from build123d import *
from OCP.BRepFilletAPI import BRepFilletAPI_MakeFillet

# Parameters (mm, degrees)
SKETCH1_W           = 55
SKETCH1_H           = 30
BOSS_EXTRUDE1_DEPTH = 3
CUT_EXTRUDE1_DEPTH  = 32.468237955
SKETCH3_W           = 6.4
SKETCH3_H           = 2
CUT_EXTRUDE2_DEPTH  = 32.468237955
SKETCH4_W           = 20.5
SKETCH4_H           = 16
CUT_EXTRUDE3_DEPTH  = 32.468237955
FILLET1_R1          = 3
FILLET1_R2          = 2.5
FILLET1_R3          = 2


with BuildPart() as part:
    # Sketch1 → Boss-Extrude1 (new body)
    with BuildSketch(Plane(origin=(0, 0, 0), x_dir=(1, 0, 0), z_dir=(0, 1, 0))):
        Rectangle(SKETCH1_W, SKETCH1_H)
    extrude(amount=BOSS_EXTRUDE1_DEPTH)

    # Sketch2 → Cut-Extrude1 (cut, through all)
    with BuildSketch(Plane(origin=(0, 3, 0), x_dir=(1, 0, 0), z_dir=(0, 1, 0))):
        with BuildLine():
            Line((17, -5.5), (24, -5.5))
            ThreePointArc((24, -5.5), (26.5, -8), (24, -10.5))
            Line((24, -10.5), (17, -10.5))
            ThreePointArc((17, -10.5), (14.5, -8), (17, -5.5))
        make_face()
        with BuildLine():
            Line((-17, -5.5), (-24, -5.5))
            ThreePointArc((-24, -5.5), (-26.5, -8), (-24, -10.5))
            Line((-24, -10.5), (-17, -10.5))
            ThreePointArc((-17, -10.5), (-14.5, -8), (-17, -5.5))
        make_face()
        with BuildLine():
            Line((-2, -2), (-2, 8))
            ThreePointArc((-2, 8), (0, 10), (2, 8))
            Line((2, 8), (2, -2))
            ThreePointArc((2, -2), (0, -4), (-2, -2))
        make_face()
    extrude(amount=-CUT_EXTRUDE1_DEPTH, mode=Mode.SUBTRACT)

    # Sketch3 → Cut-Extrude2 (cut, through all)
    with BuildSketch(Plane(origin=(0, 3, 0), x_dir=(1, 0, 0), z_dir=(0, 1, 0))):
        with Locations((0, 15)):
            Rectangle(SKETCH3_W, SKETCH3_H)
    extrude(amount=-CUT_EXTRUDE2_DEPTH, mode=Mode.SUBTRACT)

    # Sketch4 → Cut-Extrude3 (cut, through all)
    with BuildSketch(Plane(origin=(0, 3, 0), x_dir=(1, 0, 0), z_dir=(0, 1, 0))):
        with Locations((-17.25, 7)):
            Rectangle(SKETCH4_W, SKETCH4_H)
        with Locations((17.25, 7)):
            Rectangle(SKETCH4_W, SKETCH4_H)
    extrude(amount=-CUT_EXTRUDE3_DEPTH, mode=Mode.SUBTRACT)

    # Fillet1: one fillet with a radius per group of edges: ONE call of the kernel's fillet builder (fillet() takes one radius for all edges)
    fillet1_edges_1 = [part.edges().sort_by_distance(p)[0] for p in [
        (7, 1.5, 1),
        (-7, 1.5, 1),
    ]]
    fillet1_edges_2 = [part.edges().sort_by_distance(p)[0] for p in [
        (-27.5, 1.5, 1),
        (-27.5, 1.5, 15),
    ]]
    fillet1_edges_3 = [part.edges().sort_by_distance(p)[0] for p in [
        (27.5, 1.5, 1),
        (27.5, 1.5, 15),
        (7, 1.5, -15),
        (-7, 1.5, -15),
    ]]
    fillet1 = BRepFilletAPI_MakeFillet(part.part.solid().wrapped)
    for e in fillet1_edges_1:
        fillet1.Add(FILLET1_R1, e.wrapped)
    for e in fillet1_edges_2:
        fillet1.Add(FILLET1_R2, e.wrapped)
    for e in fillet1_edges_3:
        fillet1.Add(FILLET1_R3, e.wrapped)
    add(Compound.cast(fillet1.Shape()), mode=Mode.REPLACE)


solid = part.part
Geometry check sheet. Reference: the model listing, model coordinates, mm. A direction names the side the tool comes from. Give positions to 0.01 mm unless a question says otherwise; leave off trailing zeros. Loops run counter-clockwise (first coordinate to the right, second up) from the corner with the lowest first, then second, coordinate; pieces in that order, holes last. Notation, with made-up numbers: M 37.5,49 L 44.5,49 A24 ccw 44.5,77 Z; hole C 67,30.5 d11. An arc over 180 degrees is marked long. Answer as a JSON object with one key per item and string values. Group by question number.
Item 1: Material ranges on L1, parallel to Z at x = 17, y = 1.5; L2, parallel to X at y = 1.2, z = 9; L3, parallel to X at y = 0.35, z = -12.5, recorded low to high.
Item 2: Access from +Z, -Z, +X, -X, +Y, -Y to the whole of each face (thin tool, end or side, straight path). Record for faces 4 (the flat face through (7, 2, -7)), 5 (the cylindrical face through (-27, 2, 14)), 6 (the flat face through (2, 2, -3)), 7 (the flat face through (-18, 2, 1)).
Item 3: Gauge pin test, flat ends, axial feed: pin 1 (0.8 mm diameter, centred on y = 1, z = -14.5, fed in from -X); pin 2 (0.9 mm diameter, centred on x = -15, y = 1, fed in from -Z); pin 3 (0.9 mm diameter, centred on y = 1, z = -2.5, fed in from +X). Record the tip position at first contact, or that the pin passes through.
Item 4: Sectioned sample at B-B on y = 0.6. Give the number of separate pieces and of enclosed holes in the cut face, plus the area to 3 significant figures.
Item 5: Sectioned sample at A-A on x = 20.5. Record the boundary of the cut face in (y, z).
Item 6: Mould release check, pull along X, two halves, no side actions. Record for faces 1 (the flat face through (0, 3, 6)), 2 (the flat face through (-2, 2, -3)), 3 (the cylindrical face through (26.9, 1.52, 14.43)): pulls with the +X half, pulls with the -X half, needs draft (parallel to the pull), parting line crosses it, or undercut.
Findings below:
{
 "1": {"L1": "1 to 5.5, 10.5 to 15", "L2": "-27.5 to -26.29, -14.71 to 14.71, 26.29 to 27.5", "L3": "-7 to 7"},
 "2": {"face 4": "-Z, +X, +Y, -Y", "face 5": "+Z, -X, +Y, -Y", "face 6": "+Y, -Y", "face 7": "-Z, -X, +Y, -Y"},
 "3": {"pin 1": "x = -6.67", "pin 2": "z = 1", "pin 3": "x = 7"},
 "4": {"separate pieces": "1", "enclosed holes": "3", "area": "824 mm2"},
 "5": {"outline": "M 0,1 L 3,1 L 3,5.5 L 0,5.5 Z; M 0,10.5 L 3,10.5 L 3,15 L 0,15 Z"},
 "6": {"face 1": "needs draft", "face 2": "undercut", "face 3": "pulls with the +X half"}
}
